Design review of the part built by this model. Coordinates are the model's own, in mm. A direction names the side the tool comes from. Give positions to 0.01 mm unless a question says otherwise; leave off trailing zeros. Order: outer loops, then holes, each group sorted by start corner. A loop starts at its lowest first (then second) coordinate and runs counter-clockwise, first axis right, second up. Notation, with made-up numbers: (14.5, -7) -> (30.5, -7) arc R25 cw to (30.5, 19) -> close; hole circle Ø3 at (38, 2.25). An arc over 180 degrees is marked (long way). One line per item, written item: value.
from build123d import *

# Parameters (mm, degrees)
SKETCH022_R             = 2.1
SKETCH022_W             = 22
SKETCH022_H             = 42
PAD010_DEPTH            = 5
PAD013_DEPTH            = 3
PAD011_DEPTH            = 3
PAD012_DEPTH            = 12
SKETCH028_R             = 10
PAD014_DEPTH            = 4
SKETCH029_R             = 3.5
POCKET011_DEPTH         = 4
SKETCH026_R             = 10
PAD015_DEPTH            = 4
SKETCH025_R             = 5
POCKET012_DEPTH         = 4
FILLET002_R             = 15
BODY005_PLACEMENT_ANGLE = 90


with BuildPart() as part:
    # Sketch022 → Pad010 (new body)
    with BuildSketch(Plane.XZ):
        with BuildLine():
            Line((-11, 29), (11, 29))
            ThreePointArc((14, 26), (13.1213203436, 28.1213203436), (11, 29))
            Line((14, 26), (14, -26))
            ThreePointArc((11, -29), (13.1213203436, -28.1213203436), (14, -26))
            Line((11, -29), (-11, -29))
            ThreePointArc((-14, -26), (-13.1213203436, -28.1213203436), (-11, -29))
            Line((-14, -26), (-14, 26))
            ThreePointArc((-11, 29), (-13.1213203436, 28.1213203436), (-14, 26))
        make_face()
        with Locations((-4.5, -25.15)):
            Circle(SKETCH022_R, mode=Mode.SUBTRACT)
        with Locations((4.5, -25.15)):
            Circle(SKETCH022_R, mode=Mode.SUBTRACT)
        with Locations((-4.5, 25.15)):
            Circle(SKETCH022_R, mode=Mode.SUBTRACT)
        with Locations((4.5, 25.15)):
            Circle(SKETCH022_R, mode=Mode.SUBTRACT)
        Rectangle(SKETCH022_W, SKETCH022_H, mode=Mode.SUBTRACT)
    extrude(amount=PAD010_DEPTH)

    # Sketch023 (on Face1 of Pad010) → Pad013 (join)
    with BuildSketch(Plane(origin=(-14, 0, 0), x_dir=(0, 0, -1), z_dir=(-1, 0, 0))):
        with BuildLine():
            Line((4, 29.0287840283), (16, 29.0287840283))
            Line((16, 29.0287840283), (16, 24.1593727123))
            ThreePointArc((16, 24.1593727123), (18.3615371547, 13.5527709945), (25, 4.95))
            Line((-10, 4.95), (25, 4.95))
            ThreePointArc((-10, 4.95), (0.1245154966, 12.1966244621), (4, 24.0287840283))
            Line((4, 24.0287840283), (4, 29.0287840283))
        make_face()
    extrude(amount=-PAD013_DEPTH)

    # Sketch027 (on Face9 of Pad013) → Pad011 (join)
    with BuildSketch(Plane(origin=(14, 0, 0), x_dir=(0, 0, 1), z_dir=(1, 0, 0))):
        with BuildLine():
            Line((10, 4.95), (-25, 4.95))
            ThreePointArc((-25, 4.95), (-18.3615371547, 13.5527709945), (-16, 24.1593727123))
            Line((-16, 24.1593727123), (-16, 29.0287840283))
            Line((-16, 29.0287840283), (-4, 29.0287840283))
            Line((-4, 29.0287840283), (-4, 24.0287840283))
            ThreePointArc((-4, 24.0287840283), (-0.1245154966, 12.1966244621), (10, 4.95))
        make_face()
    extrude(amount=-PAD011_DEPTH)

    # Sketch024 (on Face31 of Pad011) → Pad012 (join)
    with BuildSketch(Plane(origin=(0, 0, -4), x_dir=(-1, 0, 0), z_dir=(0, 0, 1))):
        with BuildLine():
            Line((-29, 32), (29, 32))
            Line((29, 57), (29, 32))
            Line((33, 57), (29, 57))
            Line((33, 32), (33, 57))
            ThreePointArc((29, 28), (31.8284271247, 29.1715728753), (33, 32))
            ThreePointArc((29, 28), (18.3933982822, 23.6066017178), (14, 13))
            Line((14, 28), (14, 13))
            Line((-14, 28), (14, 28))
            Line((-14, 28), (-14, 13))
            ThreePointArc((-14, 13), (-18.3933982822, 23.6066017178), (-29, 28))
            ThreePointArc((-33, 32), (-31.8284271247, 29.1715728753), (-29, 28))
            Line((-33, 32), (-33, 57))
            Line((-33, 57), (-29, 57))
            Line((-29, 57), (-29, 32))
        make_face()
    extrude(amount=-PAD012_DEPTH)

    # Sketch028 (on Face53 of Pad012) → Pad014 (join)
    with BuildSketch(Plane(origin=(33, 0, 0), x_dir=(0, 0, 1), z_dir=(1, 0, 0))):
        with Locations((-10, 57)):
            Circle(SKETCH028_R)
    extrude(amount=-PAD014_DEPTH)

    # Sketch029 (on Face56 of Pad014) → Pocket011 (cut)
    with BuildSketch(Plane(origin=(33, 0, 0), x_dir=(0, 0, 1), z_dir=(1, 0, 0))):
        with Locations((-10, 57)):
            Circle(SKETCH029_R)
    extrude(amount=-POCKET011_DEPTH, mode=Mode.SUBTRACT)

    # Sketch026 (on Face47 of Pocket011) → Pad015 (join)
    with BuildSketch(Plane(origin=(-33, 0, 0), x_dir=(0, 0, -1), z_dir=(-1, 0, 0))):
        with Locations((10, 57)):
            Circle(SKETCH026_R)
    extrude(amount=-PAD015_DEPTH)

    # Sketch025 (on Face58 of Pad015) → Pocket012 (cut)
    with BuildSketch(Plane(origin=(-33, 0, 0), x_dir=(0, 0, -1), z_dir=(-1, 0, 0))):
        with Locations((10, 57)):
            Circle(SKETCH025_R)
    extrude(amount=-POCKET012_DEPTH, mode=Mode.SUBTRACT)

    # Fillet002
    fillet002_edges = [part.edges().sort_by_distance(p)[0] for p in [
        (-31, -49, -4),
        (31, -49, -16),
        (-31, -49, -16),
        (31, -49, -4),
    ]]
    fillet(fillet002_edges, radius=FILLET002_R)


with BuildPart() as part_1:
    # Body005 placement: moved
    add(part.part.moved(Location((0, -65.5, -132))).rotate(Axis((0, -65.5, -132), (-1, 0, 0)), BODY005_PLACEMENT_ANGLE))


solid = part_1.part
Item 1: Draft analysis for pull direction X (two halves, no side actions). For faces 4 (the cylindrical face through (31.859, -75.416, -102.797)), 5 (the flat face through (29, -76, -82)), 6 (the flat face through (0, -36.5, -130)), state which applies: pulls with the +X half, pulls with the -X half, needs draft (parallel to the pull), parting line crosses it, or undercut.
Returned:
face 4: pulls with the +X half
face 5: undercut
face 6: needs draft
Item 2: To check wall thickness, follow line 1 along Y through (x, z) = (4.5, -130.35); line 2 along X through (y, z) = (-70, -80.5); line 3 along Z through (x, y) = (32, -75). State the ranges of each line that lie inside material, in increasing order. Write a range as from..to.
Returned:
line 1: -94.5..-92.75, -88.55..-86.5, -44.5..-42.45, -38.25..-36.5
line 2: -33..-29, 29..33
line 3: -102.65..-78.46, -71.54..-65.01
Item 3: Machinability: for faces 1 (the cylindrical face through (12.52, -83.91, -118.55)), 2 (the flat face through (0, -90, -127)), 3 (the flat face through (0, -44, -127)), which of the approach directions +Z, -Z, +X, -X, +Y, -Y give a long, thin tool a straight path to every point of the face, cutting with its end or side? Answer none if there is none.
Returned:
face 1: +Z, +X, -X, -Y
face 2: +Z, -Y
face 3: +Z, +X, -X, +Y
Item 4: Add section D-D on z = -94.5. Give the boundary of the cut face in (x, y).
Returned:
outline: (-33, -81.5) -> (-29, -81.5) -> (-29, -69.5) -> (-33, -69.5) -> close; (29, -81.5) -> (33, -81.5) -> (33, -69.5) -> (29, -69.5) -> close
Item 5: Clearance check with flat-ended pins moving along their axes: P1, Ø12, axis at y = -64.5, z = -114, coming from the -X side; P2, Ø8, axis at x = -21.5, y = -80, coming from the +Z side; P3, Ø12, axis at x = -23, y = -47, coming from the +Z side; P4, Ø3.5, axis at x = -4.5, y = -75, coming from the -Z side. State where each tip first meets the part, or that it passes through.
Returned:
P1: x = -16.52
P2: z = -100
P3: through
P4: z = -104
Item 6: Add section B-B on x = 7.5. Give the boundary of the cut face in (y, z).
Returned:
outline: (-94.5, -132) -> (-86.5, -132) -> (-86.5, -127) -> (-94.5, -127) -> close; (-81.5, -104) -> (-69.5, -104) -> (-69.5, -100) -> (-81.5, -100) -> close; (-44.5, -132) -> (-36.5, -132) -> (-36.5, -127) -> (-44.5, -127) -> close
Item 7: Add section A-A on z = -75. Give the boundary of the cut face in (x, y), plus the area to 3 significant figures.
Returned:
outline: (-33, -85.5) -> (-29, -85.5) -> (-29, -80.5) -> (-33, -80.5) -> close; (-33, -70.5) -> (-29, -70.5) -> (-29, -65.5) -> (-33, -65.5) -> close; (29, -85.5) -> (33, -85.5) -> (33, -79) -> (29, -79) -> close; (29, -72) -> (33, -72) -> (33, -65.5) -> (29, -65.5) -> close
area: 92.0 mm²
Item 8: Add section C-C on y = -75.5. Give the boundary of the cut face in (x, z).
Returned:
outline: (-33, -100) arc R4 ccw to (-29, -104) arc R15 cw to (-14, -119) -> (-14, -132) -> (-11, -132) -> (-11, -104) -> (11, -104) -> (11, -132) -> (14, -132) -> (14, -119) arc R15 cw to (29, -104) arc R4 ccw to (33, -100) -> (33, -78.5) -> (29, -78.5) -> (29, -100) -> (-29, -100) -> (-29, -80) -> (-33, -80) -> close; (-33, -70) -> (-29, -70) -> (-29, -65) -> (-33, -65) -> close; (29, -71.5) -> (33, -71.5) -> (33, -65) -> (29, -65) -> close
